from build123d import *

# Parameters (mm, degrees)
SKETCH1_W           = 165
SKETCH1_H           = 76
BOSS_EXTRUDE1_DEPTH = 1.5
CUT_EXTRUDE1_REACH  = 140.731
SKETCH2_R           = 1.5
SKETCH3_W           = 12
SKETCH3_H           = 40
BOSS_EXTRUDE2_DEPTH = 8
SKETCH4_W           = 50
SKETCH4_H           = 50
BOSS_EXTRUDE3_DEPTH = 32
SKETCH5_W           = 30
SKETCH5_H           = 10
BOSS_EXTRUDE4_DEPTH = 10
BOSS_EXTRUDE5_DEPTH = 25
FILLET2_R           = 5
SKETCH8_R           = 4.5
SKETCH8_R_2         = 0.75
CUT_EXTRUDE2_DEPTH  = 6
CUT_EXTRUDE3_DEPTH  = 3


with BuildPart() as part:
    # Sketch1 → Boss-Extrude1 (new body)
    with BuildSketch(Plane.XY):
        with Locations((47.261306533, -11.052763819)):
            Rectangle(SKETCH1_W, SKETCH1_H)
    extrude(amount=BOSS_EXTRUDE1_DEPTH)

    # Sketch2 → Cut-Extrude1 (cut, up to next)
    with BuildSketch(Plane.XY.offset(1.5), mode=Mode.PRIVATE) as cut_extrude1_sk1:
        with Locations((124.761306533, 21.947236181)):
            Circle(SKETCH2_R)
    cut_extrude1_tool1 = extrude(cut_extrude1_sk1.sketch, amount=-CUT_EXTRUDE1_REACH, mode=Mode.PRIVATE) & part.part
    # Sketch2 → Cut-Extrude1 (cut, up to next)
    with BuildSketch(Plane.XY.offset(1.5), mode=Mode.PRIVATE) as cut_extrude1_sk2:
        with Locations((124.761306533, -44.052763819)):
            Circle(SKETCH2_R)
    cut_extrude1_tool2 = extrude(cut_extrude1_sk2.sketch, amount=-CUT_EXTRUDE1_REACH, mode=Mode.PRIVATE) & part.part
    # Sketch2 → Cut-Extrude1 (cut, up to next)
    with BuildSketch(Plane.XY.offset(1.5), mode=Mode.PRIVATE) as cut_extrude1_sk3:
        with Locations((-30.238693467, -44.052763819)):
            Circle(SKETCH2_R)
    cut_extrude1_tool3 = extrude(cut_extrude1_sk3.sketch, amount=-CUT_EXTRUDE1_REACH, mode=Mode.PRIVATE) & part.part
    # Sketch2 → Cut-Extrude1 (cut, up to next)
    with BuildSketch(Plane.XY.offset(1.5), mode=Mode.PRIVATE) as cut_extrude1_sk4:
        with Locations((-30.238693467, 21.947236181)):
            Circle(SKETCH2_R)
    cut_extrude1_tool4 = extrude(cut_extrude1_sk4.sketch, amount=-CUT_EXTRUDE1_REACH, mode=Mode.PRIVATE) & part.part
    add(cut_extrude1_tool1.solids().sort_by_distance((124.761307, 21.947236, 1.5))[0], mode=Mode.SUBTRACT)
    add(cut_extrude1_tool2.solids().sort_by_distance((124.761307, -44.052764, 1.5))[0], mode=Mode.SUBTRACT)
    add(cut_extrude1_tool3.solids().sort_by_distance((-30.238693, -44.052764, 1.5))[0], mode=Mode.SUBTRACT)
    add(cut_extrude1_tool4.solids().sort_by_distance((-30.238693, 21.947236, 1.5))[0], mode=Mode.SUBTRACT)

    # Sketch3 → Boss-Extrude2 (add)
    with BuildSketch(Plane(origin=(0, 0, 0), x_dir=(-1, 0, 0), z_dir=(0, 0, -1))):
        with Locations((-123.761306533, -7.052763819)):
            Rectangle(SKETCH3_W, SKETCH3_H)
    extrude(amount=BOSS_EXTRUDE2_DEPTH)

    # Sketch4 → Boss-Extrude3 (add)
    with BuildSketch(Plane(origin=(0, 0, 0), x_dir=(-1, 0, 0), z_dir=(0, 0, -1))):
        with Locations((-94.761306533, -14.052763819)):
            Rectangle(SKETCH4_W, SKETCH4_H)
    extrude(amount=BOSS_EXTRUDE3_DEPTH)

    # Sketch5 → Boss-Extrude4 (add)
    with BuildSketch(Plane(origin=(0, 0, 0), x_dir=(-1, 0, 0), z_dir=(0, 0, -1))):
        with Locations((35.238693467, 10.947236181)):
            Rectangle(SKETCH5_W, SKETCH5_H)
        with Locations((35.238693467, -15.552763819)):
            Rectangle(SKETCH5_W, SKETCH5_H)
    extrude(amount=BOSS_EXTRUDE4_DEPTH)

    # Sketch6 → Boss-Extrude5 (add)
    with BuildSketch(Plane(origin=(0, 0, 0), x_dir=(-1, 0, 0), z_dir=(0, 0, -1))):
        Polygon((0.079164122, 4.887423166), (-1.341039882, 7.229369498), (-3.636731908, 8.72318681), (-6.353221994, 9.073006263), (-8.952475964, 8.209541823), (-10.919679691, 6.303813212), (-11.86520435, 3.733273355), (-11.601777188, 1.007049196), (-10.181573183, -1.334897137), (-7.885881157, -2.828714449), (-5.169391071, -3.178533901), (-2.570137101, -2.315069461), (-0.602933374, -0.409340851), (0.342591285, 2.161199006), align=None)
    extrude(amount=BOSS_EXTRUDE5_DEPTH)

    # Fillet2
    fillet2_edges = [part.edges().sort_by_distance(p)[0] for p in [
        (-42.738693467, 5.947236181, 0),
        (-42.738693467, 15.947236181, 0),
        (-35.238693467, 15.947236181, -10),
        (-35.238693467, 5.947236181, -10),
        (-42.738693467, -20.552763819, 0),
        (-42.738693467, -10.552763819, 0),
        (-35.238693467, -10.552763819, -10),
        (-35.238693467, -20.552763819, -10),
    ]]
    fillet(fillet2_edges, radius=FILLET2_R - 0.0001)  # a hair under: the kernel refuses the full size

    # Sketch8 → Cut-Extrude2 (cut)
    # profile 1 of 2: a face of its own
    with BuildSketch(Plane.ZY.offset(50.238693467)):
        with Locations((-5, -15.552763819)):
            Circle(SKETCH8_R)
        with Locations((-5, -15.552763819)):
            Circle(SKETCH8_R_2, mode=Mode.SUBTRACT)
    # profile 2 of 2: a face of its own
    with BuildSketch(Plane.ZY.offset(50.238693467)):
        with Locations((-5, 10.947236181)):
            Circle(SKETCH8_R)
        with Locations((-5, 10.947236181)):
            Circle(SKETCH8_R_2, mode=Mode.SUBTRACT)
    extrude(amount=-CUT_EXTRUDE2_DEPTH, mode=Mode.SUBTRACT)

    # Sketch10 → Cut-Extrude3 (cut)
    with BuildSketch(Plane(origin=(0, 0, -25), x_dir=(-1, 0, 0), z_dir=(0, 0, -1))):
        Polygon((-5.761306533, 2.947236181), (-1.341039882, 7.229369498), (0.079164122, 4.887423166), align=None)
    extrude(amount=-CUT_EXTRUDE3_DEPTH, mode=Mode.SUBTRACT)


solid = part.part
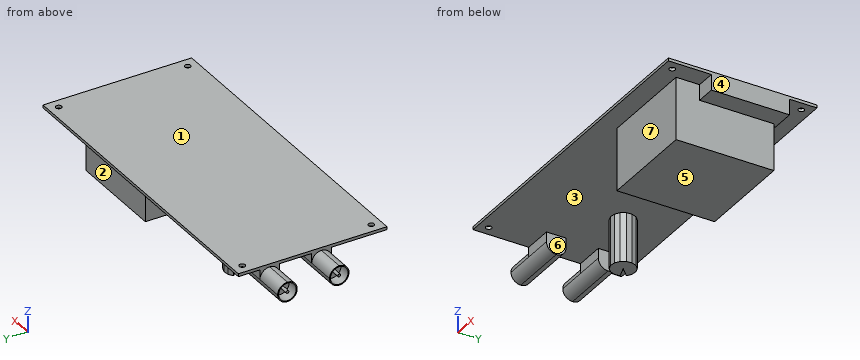
Design review of the part built by this model. Coordinates are the model's own, in mm. Face numbers are marked on the shaded views. A direction names the side the tool comes from. Coordinates: 2 decimals unless noted, no trailing zeros. Write each loop counter-clockwise with the first axis right and the second up, starting at its lowest first coordinate (ties: lowest second). Pieces come first, ordered by that corner, then holes. Notation, with made-up numbers: (20.25, 61) -> (37.25, 61) arc R31 cw to (37.25, 92) -> close; hole circle Ø10 at (44.25, -29). An arc over 180 degrees is marked (long way). Write each question's results on one line, items separated by ' | '. Start each with the question number.
(1) Take a section at D-D on y = -13. Write out the cut boundary in (x, z), and give its area (3 significant figures).
(2) Take a section at A-A on z = -18. Write out the cut boundary in (x, y), and give its area (3 significant figures).
(3) The part is to be moulded in two halves that separate along X. For the marked faces 1, 2, 3 and 4, say which applies: pulls with the +X half, pulls with the -X half, needs draft (parallel to the pull), parting line crosses it, or undercut.
(4) Take a section at B-B on y = -25. Write out the cut boundary in (x, z).
(5) For line 1 along Y through (x, z) = (-46, -5); line 2 along X through (y, z) = (-17.5, -7); line 3 along Y through (x, z) = (-20.5, -4), list the stretches that pass through material, from the lowest coordinate up. Write a range as from..to.
(6) Take a section at C-C on x = 64. Write out the cut boundary in (y, z).
(7) Tool access review of the marked faces 5, 6 and 7: name each direction out of +Z, -Z, +X, -X, +Y, -Y from which nothing blocks a thin tool from reaching the whole face with its end or side.
(8) Clearance check with flat-ended pins moving along their axes: P1, Ø16, axis at x = 87, z = -22.5, coming from the +Y side; P2, Ø2, axis at x = 35, y = -8, coming from the -Z side; P3, Ø2.5, axis at x = 124.76, y = 21.95, coming from the -Z side; P4, Ø6.5, axis at x = 122, z = -5, coming from the +Y side. State where each tip first meets the part, or that it passes through.
Results found:
1) outline: (-50.24, -9.3) -> (-20.24, -9.3) -> (-20.24, 0) -> (69.76, 0) -> (69.76, -32) -> (119.76, -32) -> (119.76, -8) -> (129.76, -8) -> (129.76, 1.5) -> (-35.24, 1.5) -> (-35.24, -0.7) -> (-50.24, -0.7) -> (-50.24, -1.29) -> (-44.24, -1.29) -> (-44.24, -8.71) -> (-50.24, -8.71) -> close | area: 2,150 mm2
2) outline: (-0.34, 2.16) -> (0.6, -0.41) -> (2.57, -2.32) -> (5.17, -3.18) -> (7.89, -2.83) -> (10.18, -1.33) -> (11.6, 1.01) -> (11.87, 3.73) -> (10.92, 6.3) -> (8.95, 8.21) -> (6.35, 9.07) -> (3.64, 8.72) -> (1.34, 7.23) -> (-0.08, 4.89) -> close; (69.76, -39.05) -> (119.76, -39.05) -> (119.76, 10.95) -> (69.76, 10.95) -> close | area: 2,620 mm2
3) face 1: needs draft | face 2: undercut | face 3: undercut | face 4: pulls with the +X half
4) outline: (-35.24, 0) -> (69.76, 0) -> (69.76, -32) -> (119.76, -32) -> (119.76, -8) -> (129.76, -8) -> (129.76, 1.5) -> (-35.24, 1.5) -> close
5) line 1: y = -20.55..-20.05, -16.3..-14.8, -11.05..-10.55, 5.95..6.45, 10.2..11.7, 15.45..15.95 | line 2: x = -44.24..-20.24, 69.76..129.76 | line 3: y = -20.55..-10.55, 5.95..15.95
6) outline: (-49.05, 0) -> (26.95, 0) -> (26.95, 1.5) -> (-49.05, 1.5) -> close
7) face 5: -Z, +X, -X, +Y, -Y | face 6: -Z, +Y, -Y | face 7: -Z, +X, -X, -Y
8) P1: stops at y = 10.95 | P2: stops at z = 0 | P3: passes through | P4: stops at y = 12.95
